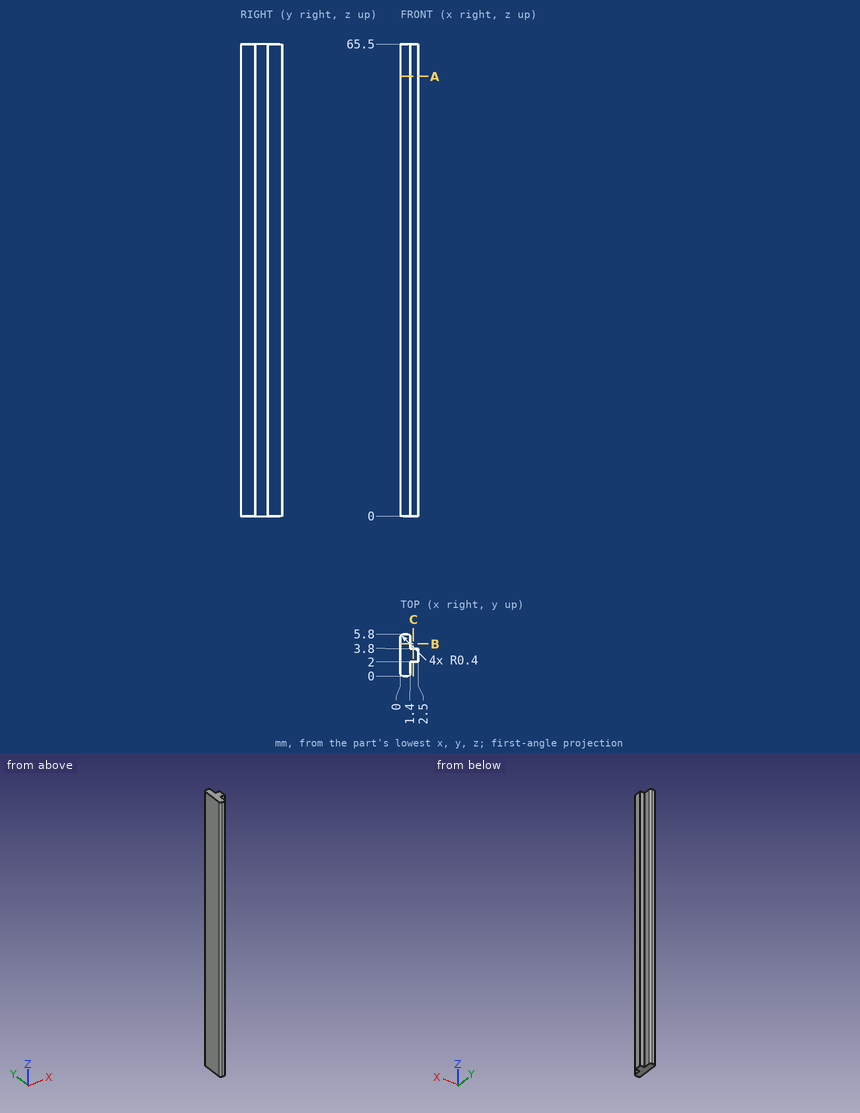
The figure shows three views and two pictorial views of one solid part (mm, origin at its lowest corner). Answer the questions. Round coordinates to 2 decimals unless told otherwise and drop trailing zeros. Order: outer loops, then holes, each group sorted by start corner. A loop starts at its lowest first (then second) coordinate and runs counter-clockwise, first axis right, second up. Notation, with made-up numbers: (33, 75) - (42, 75) arc R14 ccw to (42, 92) - close; hole circle Ø4 at (22, 39). An arc over 180 degrees is marked (long way). Write item = value, one per line. Start each with the question number.
1) Given pin 1 (1.5 mm diameter, centred on y = 1, z = 20.5, fed in from +X); pin 2 (1.5 mm diameter, centred on x = 2, z = 25, fed in from -Y); pin 3 (0.6 mm diameter, centred on x = 2, z = 18, fed in from +Y), each flat-ended and moving along its own axis, determine where each tip first touches the part or whether it passes through.
2) Section A-A, the plane z = 61 is taken. Write down the section's boundary in (x, y).
3) Section C-C, the plane x = 1.8 is taken. Write down the section's boundary in (y, z).
4) Section B-B, the plane y = 4.45 is taken. Write down the section's boundary in (x, z).
5) Straight lines are drawn through the part: L1, parallel to Y at x = 2.1, z = 26; L2, parallel to Y at x = 1.1, z = 16; L3, parallel to X at y = 0.5, z = 55. For each, find the intervals that lie inside material, in ascending order.
Results list:
q1.pin_1 = 1.4
q1.pin_2 = 0.09
q1.pin_3 = 3.8
q2.outline = (0, 0.4) arc R0.4 ccw to (0.4, 0) - (1, 0) arc R0.4 ccw to (1.4, 0.4) - (1.4, 2) - (2.5, 2) - (2.5, 3.8) - (1.4, 3.8) - (1.4, 5.4) arc R0.4 ccw to (1, 5.8) - (0.4, 5.8) arc R0.4 ccw to (0, 5.4) - close
q3.outline = (2, 0) - (3.8, 0) - (3.8, 65.5) - (2, 65.5) - close
q4.outline = (0, 0) - (1.4, 0) - (1.4, 65.5) - (0, 65.5) - close
q5.L1 = 2 to 3.8
q5.L2 = 0.01 to 5.79
q5.L3 = 0 to 1.4
